Source: CAD feature listing. Evaluate the final solid. Frame: model axes, mm. A direction names the side the tool comes from. Give positions to 0.01 mm unless a question says otherwise; leave off trailing zeros. Order: outer loops, then holes, each group sorted by start corner. A loop starts at its lowest first (then second) coordinate and runs counter-clockwise, first axis right, second up. Notation, with made-up numbers: (-31, -23) - (20, -23) arc R10 cw to (20, -18) - close; hole circle Ø9 at (31, -9.5). An arc over 180 degrees is marked (long way). Write each question's results on one line, items separated by ' | '. Start each with the question number.
Item 1: Contact query for flat-ended pins moving along their axis: pin 1 Ø2 at (y, z) = (0, 4) entering from +X; pin 2 Ø2.5 at (x, z) = (-2.5, 2.5) entering from -Y; pin 3 Ø3 at (x, z) = (10, 3.5) entering from +Y. Output: stop coordinate, or through.
Item 2: Section C-C on x = 35. Output: boundary loops of the cut face in (y, z).
Item 3: Set-up query: faces 1 (the flat face through (7, 12.5, 2)), 2 (the flat face through (-6.862, 0, 4)). Return all of +Z, -Z, +X, -X, +Y, -Y with unobstructed straight access to the full face (end or side cutting, diameter ignored); none if empty.
Item 4: Section D-D on x = 25. Output: boundary loops of the cut face in (y, z), and give its area (3 significant figures).
Item 5: Mould query, pull axis X, two halves, no side actions, for faces 3 (the flat face through (-21, 8.032, 4)), 4 (the flat face through (-1, 0, 0)). Classes: released by +X, released by -X, zero draft, split by the parting line, or undercut.
Item 6: Section A-A on y = -15.5. Output: boundary loops of the cut face in (x, z).
Item 7: Line query: line 1 along Y through (x, z) = (24.5, 3.7); line 2 along X through (y, z) = (-20.5, 3.7); line 3 along Z through (x, y) = (27.5, 22). Output: solid intervals per line, ascending.
Item 8: Section B-B on x = -8.5. Output: boundary loops of the cut face in (y, z), and give its area (3 significant figures).
```python
from build123d import *

# Parameters (mm, degrees)
F1_DEPTH = 3
F3_DEPTH = 2
F5_DEPTH = 2
F6_DEPTH = 2


# Not quite as in the source:
# - a feature of the source that left no trace in its solid (it failed there, or was rolled back) is left out


with BuildPart() as f1:
    # F0 (on Top) → F1 (new body)
    with BuildSketch(Plane.XY):
        with BuildLine():
            Line((-3, 12.5), (-10, 12.5))
            ThreePointArc((-10, 12.5), (-32.0931858273, 25.7169101843), (-33.2915619759, 0))
            ThreePointArc((-33.2915619759, 0), (-32.0931858273, -25.7169101843), (-10, -12.5))
            Line((-10, -12.5), (10, -12.5))
            ThreePointArc((10, -12.5), (32.0931858273, -25.7169101843), (33.2915619759, 0))
            ThreePointArc((33.2915619759, 0), (32.0931858273, 25.7169101843), (10, 12.5))
            Line((10, 12.5), (3, 12.5))
            ThreePointArc((3, 12.5), (0, 15.5), (-3, 12.5))
        make_face()
    extrude(amount=F1_DEPTH)

    # F2 (on face) → F3 (join)
    with BuildSketch(Plane.XY.offset(3)):
        with BuildLine():
            ThreePointArc((33.2915619759, 0), (32.0931858273, 25.7169101843), (10, 12.5))
            Line((10, 12.5), (3, 12.5))
            ThreePointArc((3, 12.5), (0, 15.5), (-3, 12.5))
            Line((-3, 12.5), (-10, 12.5))
            ThreePointArc((-10, 12.5), (-32.0931858273, 25.7169101843), (-33.2915619759, 0))
            ThreePointArc((-33.2915619759, 0), (-32.0931858273, -25.7169101843), (-10, -12.5))
            Line((-10, -12.5), (10, -12.5))
            ThreePointArc((10, -12.5), (32.0931858273, -25.7169101843), (33.2915619759, 0))
        make_face()
        with BuildLine():
            ThreePointArc((-10.6125054301, -11.9), (-31.9642656137, -25.1039281362), (-32.1491258207, 0))
            ThreePointArc((-32.1491258207, 0), (-31.9642656137, 25.1039281362), (-10.6125054301, 11.9))
            Line((-10.6125054301, 11.9), (0, 11.9))
            Line((0, 11.9), (10.6125054301, 11.9))
            ThreePointArc((10.6125054301, 11.9), (31.9642656137, 25.1039281362), (32.1491258207, 0))
            ThreePointArc((32.1491258207, 0), (31.9642656137, -25.1039281362), (10.6125054301, -11.9))
            Line((10.6125054301, -11.9), (-10.6125054301, -11.9))
        make_face(mode=Mode.SUBTRACT)
    extrude(amount=F3_DEPTH)

    # F4 (on face) → F5 (join)
    with BuildSketch(Plane.XY.offset(3)):
        with BuildLine():
            Line((-20.0455729167, 4.8259567143), (-16.46484375, -6.8407099524))
            Line((-16.46484375, -6.8407099524), (-13.57421875, -6.8407099524))
            Line((-13.57421875, -6.8407099524), (-9.7395833333, 4.8064254643))
            Line((-9.7395833333, 4.8064254643), (-9.6484375, 4.8064254643))
            add(Edge.make_bspline(
                [(-9.78515625, 1.3493942143), (-9.7688802083, 2.000435881), (-9.6484375, 4.8064254643)],
                knots=[0, 0, 0, 1, 1, 1], degree=2))
            add(Edge.make_bspline(
                [(-9.8014322917, 0.2003056726), (-9.8014322917, 0.6983525476), (-9.78515625, 1.3493942143)],
                knots=[0, 0, 0, 1, 1, 1], degree=2))
            Line((-9.8014322917, 0.2003056726), (-9.8014322917, -6.8407099524))
            Line((-9.8014322917, -6.8407099524), (-6.8619791667, -6.8407099524))
            Line((-6.8619791667, -6.8407099524), (-6.8619791667, 8.0323369226))
            Line((-6.8619791667, 8.0323369226), (-11.15234375, 8.0323369226))
            Line((-11.15234375, 8.0323369226), (-14.8860677083, -3.341360994))
            Line((-14.8860677083, -3.341360994), (-14.9479166667, -3.341360994))
            Line((-14.9479166667, -3.341360994), (-18.466796875, 8.0323369226))
            Line((-18.466796875, 8.0323369226), (-22.7604166667, 8.0323369226))
            Line((-22.7604166667, 8.0323369226), (-22.7604166667, -6.8407099524))
            Line((-22.7604166667, -6.8407099524), (-19.94140625, -6.8407099524))
            Line((-19.94140625, -6.8407099524), (-19.94140625, 0.076607756))
            add(Edge.make_bspline(
                [(-20.13671875, 4.8259567143), (-19.94140625, 1.268014006), (-19.94140625, 0.076607756)],
                knots=[0, 0, 0, 1, 1, 1], degree=2))
            Line((-20.13671875, 4.8259567143), (-20.0455729167, 4.8259567143))
        make_face()
    extrude(amount=F5_DEPTH)

    # F4 (on face) → F6 (join)
    with BuildSketch(Plane.XY.offset(3)):
        Polygon((4.9088541667, -3.2990432857), (5.986328125, -6.8407099524), (9.384765625, -6.8407099524), (4.1145833333, 8.094185881), (0.2604166667, 8.094185881), (-4.990234375, -6.8407099524), (-1.591796875, -6.8407099524), (-0.5143229167, -3.2990432857), align=None)
        with BuildLine():
            add(Edge.make_bspline(
                [(4.1536458333, -0.655814119), (2.6595052083, 4.1553837976), (2.470703125, 4.7868942143)],
                knots=[0, 0, 0, 1, 1, 1], degree=2))
            Line((4.1536458333, -0.655814119), (0.2799479167, -0.655814119))
            add(Edge.make_bspline(
                [(2.2005208333, 5.7829879643), (1.865234375, 4.480904631), (0.2799479167, -0.655814119)],
                knots=[0, 0, 0, 1, 1, 1], degree=2))
            add(Edge.make_bspline(
                [(2.470703125, 4.7868942143), (2.2819010417, 5.418404631), (2.2005208333, 5.7829879643)],
                knots=[0, 0, 0, 1, 1, 1], degree=2))
        make_face(mode=Mode.SUBTRACT)
    extrude(amount=F6_DEPTH)


solid = f1.part
```
Evaluation:
1) pin 1: stops at x = 34.63 | pin 2: stops at y = -12.5 | pin 3: stops at y = 19.04
2) outline: (-23.68, 0) - (-1.32, 0) - (-1.32, 5) - (-2.14, 5) - (-2.14, 3) - (-22.86, 3) - (-22.86, 5) - (-23.68, 5) - close; (1.32, 0) - (23.68, 0) - (23.68, 5) - (22.86, 5) - (22.86, 3) - (2.14, 3) - (2.14, 5) - (1.32, 5) - close
3) face 1: +Z, -Z, +Y | face 2: +Z
4) outline: (-27.5, 0) - (27.5, 0) - (27.5, 5) - (26.9, 5) - (26.9, 3) - (-26.9, 3) - (-26.9, 5) - (-27.5, 5) - close | area: 167 mm^2
5) face 3: undercut | face 4: zero draft
6) outline: (-39.7, 0) - (-10.3, 0) - (-10.3, 5) - (-10.92, 5) - (-10.92, 3) - (-39.08, 3) - (-39.08, 5) - (-39.7, 5) - close; (10.3, 0) - (39.7, 0) - (39.7, 5) - (39.08, 5) - (39.08, 3) - (10.92, 3) - (10.92, 5) - (10.3, 5) - close
7) line 1: y = -27.49 to -26.89, 26.89 to 27.49 | line 2: x = -37.69 to -36.97, -13.03 to -12.31, 12.31 to 13.03, 36.97 to 37.69 | line 3: z = 0 to 3
8) outline: (-12.5, 0) - (12.5, 0) - (12.5, 5) - (11.9, 5) - (11.9, 3) - (8.03, 3) - (8.03, 5) - (-6.84, 5) - (-6.84, 3) - (-11.9, 3) - (-11.9, 5) - (-12.5, 5) - close | area: 107 mm^2
